from build123d import *

# Parameters (mm, degrees)
F0_R     = 22.5
F0_R_2   = 12.5
F1_DEPTH = 2
F2_R     = 15
F2_R_2   = 12.5
F3_DEPTH = 50


# Not quite as in the source:
# - a fillet or chamfer that OpenCascade refuses, or shapes differently, is made with other operations: its cross-section is extruded or revolved along the edge and cut away or added


with BuildPart() as f1:
    # F0 (on Top) → F1 (new body)
    with BuildSketch(Plane.XY):
        Circle(F0_R)
        Circle(F0_R_2, mode=Mode.SUBTRACT)
    extrude(amount=F1_DEPTH)

    # F2 (on face) → F3 (join)
    with BuildSketch(Plane.XY.offset(2)):
        Circle(F2_R)
        Circle(F2_R_2, mode=Mode.SUBTRACT)
    extrude(amount=F3_DEPTH)

    # F4: fillet of radius 3 on 2 edges, made by hand

    # F4_s1 → F4_t2 (revolve, cut)
    with BuildSketch(Plane.XZ):
        with BuildLine():
            ThreePointArc((12.5, 3), (13.3786796564, 0.8786796564), (15.5, 0))
            Line((15.5, 0), (12.5, 0))
            Line((12.5, 0), (12.5, 3))
        make_face()
    revolve(axis=Axis((0, 0, 0), (0, 0, 1)), mode=Mode.SUBTRACT)

    # F4_s3 → F4_t4 (revolve, cut)
    with BuildSketch(Plane.XZ):
        with BuildLine():
            ThreePointArc((15, 52), (13.2087121525, 50.9784517816), (12.5, 49.0419601084))
            Line((12.5, 49.0419601084), (12.5, 52))
            Line((12.5, 52), (15, 52))
        make_face()
    revolve(axis=Axis((0, 0, 52), (0, 0, 1)), mode=Mode.SUBTRACT)


solid = f1.part
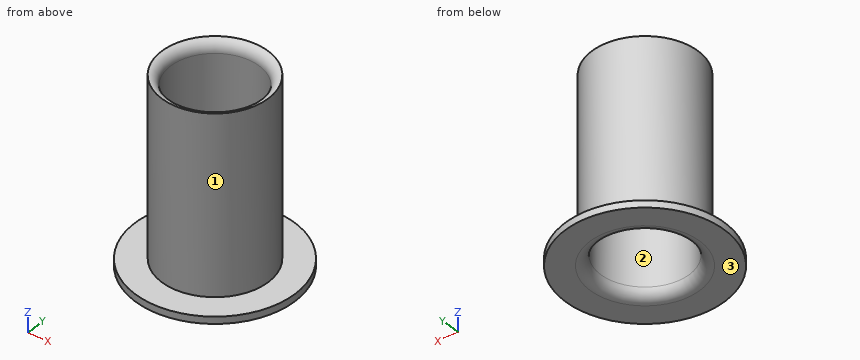
The listing builds one solid part. Answer for the finished solid, in the listing's coordinates (mm). Face numbers are marked on the shaded views. Give positions to 0.01 mm unless a question says otherwise; leave off trailing zeros. Order: outer loops, then holes, each group sorted by start corner. A loop starts at its lowest first (then second) coordinate and runs counter-clockwise, first axis right, second up. Notation, with made-up numbers: (88, 35) - (93, 35) arc R22 cw to (93, 56) - close; hole circle Ø6 at (-13, 28). An arc over 180 degrees is marked (long way). One line per item, written item: value. Start each with the question number.
1) A cutting plane is placed at A-A on y = 0. Give the vertices of the cut face in (x, z).
2) Find the intervals of material crossed by L1, parallel to Y at x = 0.5, z = 3; L2, parallel to Z at x = -11, y = -17.5; L3, parallel to Y at x = -9, z = 3.5, in increasing order.
3) A cutting plane is placed at C-C on z = 48. Give the vertices of the cut face in (x, y), then the cut area to 3 significant figures.
4) The mould has two halves that part along Y. Classify the marked faces 1, 2 and 3: released by +Y, released by -Y, zero draft, split by the parting line, or undercut.
5) A cutting plane is placed at D-D on y = -16.5. Give the vertices of the cut face in (x, z), then the cut area to 3 significant figures.
6) Given pin 1 Ø4 at (y, z) = (-7, 29.5) entering from +X; pin 2 Ø6 at (y, z) = (-11.5, 24.5) entering from -X; pin 3 Ø6 at (y, z) = (-16, 29.5) entering from -X, each flat-ended and moving along its own axis, determine where each tip first touches the part or whether it passes through.
Answer sheet:
1. outline: (-22.5, 0) - (-15.5, 0) arc R3 ccw to (-12.5, 3) - (-12.5, 49.04) arc R3 ccw to (-15, 52) - (-15, 2) - (-22.5, 2) - close; (12.5, 3) arc R3 ccw to (15.5, 0) - (22.5, 0) - (22.5, 2) - (15, 2) - (15, 52) arc R3 ccw to (12.5, 49.04) - close
2. L1: y = -14.99 to -12.49, 12.49 to 14.99
2. L2: z = 0 to 2
2. L3: y = -12 to -8.67, 8.67 to 12
3. outline: circle Ø30 at (0, 0); hole circle Ø25 at (0, 0)
3. area: 216 mm2
4. face 1: split by the parting line
4. face 2: undercut
4. face 3: zero draft
5. outline: (-15.3, 0) - (15.3, 0) - (15.3, 2) - (-15.3, 2) - close
5. area: 61.2 mm2
6. pin 1: stops at x = 14.14
6. pin 2: stops at x = -12.36
6. pin 3: stops at x = -7.48
